Part model, mm, in its own coordinate system. A direction names the side the tool comes from. Round coordinates to 2 decimals unless told otherwise and drop trailing zeros. Loops run counter-clockwise (first coordinate to the right, second up) from the corner with the lowest first, then second, coordinate; pieces in that order, holes last.
(1) Probe probe 1 along Z at (x, y) = (7.75, 3.5); probe 2 along X at (y, z) = (5, 2.5); probe 3 along X at (y, z) = (2.75, 8.25). List the from-to ranges inside material, lowest first.
(2) Cut at A-A on z = 13.75. List the corners of the cut face in (x, y), then the cut area to 3 significant figures.
(3) Tool access for faces 5 (the face through (10.1, 4.9, 5.4)), 6 (the face through (5.9, 3, 10)): list every direction of +Z, -Z, +X, -X, +Y, -Y with a clear straight run to the whole face (end or side of a thin tool).
(4) Cut at C-C on y = 2. List the corners of the cut face in (x, z).
(5) Mould opens along Z. For faces 1 (the face through (14.3, 0, 9.9)), 2 (the face through (14.1, 1, 10)), 3 (the face through (5, 3, 0)), 4 (the face through (9, 3, 5.9)) say: +Z half, -Z half, draft (parallel to the pull), parting line (faces both ways), or undercut.
(6) Cut at D-D on z = 3.25. List the corners of the cut face in (x, y).
(7) Cut at B-B on x = 7. List the corners of the cut face in (y, z) (3 decimals), then the cut area to 3 significant figures.
(8) Flat gauge pin, fed straight in: pin 1 (3.5 mm diameter, centred on y = 2.5, z = 12, fed in from +X). Where does the tip first touch, or does it go through?
from build123d import *

# Parameters (mm, degrees)
SALIENTE_EXTRUIR1_DEPTH = 20
CROQUIS2_W              = 8.2
CROQUIS2_H              = 8.2
CORTAR_EXTRUIR1_DEPTH   = 20


with BuildPart() as part:
    # Croquis1 → Saliente-Extruir1 (new body)
    with BuildSketch(Plane.XY):
        Polygon((0, 0), (20, 0), (0, 9.9), align=None)
    extrude(amount=SALIENTE_EXTRUIR1_DEPTH)

    # Croquis2 → Cortar-Extruir1 (cut)
    with BuildSketch(Plane.XZ):
        with Locations((10, 10)):
            Rectangle(CROQUIS2_W, CROQUIS2_H)
    extrude(amount=-CORTAR_EXTRUIR1_DEPTH, mode=Mode.SUBTRACT)


solid = part.part
Final values:
1. probe 1: z = 0 to 5.9, 14.1 to 20
1. probe 2: x = 0 to 9.9
1. probe 3: x = 0 to 5.9, 14.1 to 14.44
2. outline: (0, 0) - (5.9, 0) - (5.9, 6.98) - (0, 9.9) - close; (14.1, 0) - (20, 0) - (14.1, 2.92) - close
2. area: 58.4 mm2
3. face 5: +Z, -Z, +X, +Y
3. face 6: +Y, -Y
4. outline: (0, 0) - (15.96, 0) - (15.96, 20) - (0, 20) - close; hole (5.9, 5.9) - (14.1, 5.9) - (14.1, 14.1) - (5.9, 14.1) - close
5. face 1: draft
5. face 2: undercut
5. face 3: -Z half
5. face 4: undercut
6. outline: (0, 0) - (20, 0) - (0, 9.9) - close
7. outline: (0, 0) - (6.435, 0) - (6.435, 5.9) - (0, 5.9) - close; (0, 14.1) - (6.435, 14.1) - (6.435, 20) - (0, 20) - close
7. area: 75.9 mm2
8. pin 1: stops at x = 18.48
